from build123d import *

# Parameters (mm, degrees)
F0_R     = 22
F1_DEPTH = 6
F2_R     = 1.75
F3_DEPTH = 6.001
F4_R     = 5.5
F5_DEPTH = 4
F6_R     = 9
F7_DEPTH = 40
F8_R     = 5
F9_DEPTH = 35


with BuildPart() as f1:
    # F0 (on Front) → F1 (new body)
    with BuildSketch(Plane.XZ):
        Circle(F0_R)
    extrude(amount=F1_DEPTH)

    # F2 (on face) → F3 (cut, through all)
    with BuildSketch(Plane.XZ.offset(6)):
        with Locations((-8.301622, -8.665049)):
            Circle(F2_R)
        with Locations((8.665049, -8.301622)):
            Circle(F2_R)
        with Locations((-8.665049, 8.301622)):
            Circle(F2_R)
        with Locations((7.944154, 8.99391)):
            Circle(F2_R)
    extrude(amount=-F3_DEPTH, mode=Mode.SUBTRACT)

    # F4 (on face) → F5 (cut)
    with BuildSketch(Plane.XZ.offset(6)):
        Circle(F4_R)
    extrude(amount=-F5_DEPTH, mode=Mode.SUBTRACT)

    # F6 (on face) → F7 (join)
    with BuildSketch(Plane(origin=(0, 0, 0), x_dir=(-1, 0, 0), z_dir=(0, 1, 0))):
        Circle(F6_R)
    extrude(amount=F7_DEPTH)

    # F8 (on face) → F9 (cut)
    with BuildSketch(Plane(origin=(0, 40, 0), x_dir=(-1, 0, 0), z_dir=(0, 1, 0))):
        Circle(F8_R)
    extrude(amount=-F9_DEPTH, mode=Mode.SUBTRACT)


solid = f1.part
Source: CAD feature listing. Evaluate the final solid. Frame: model axes, mm. A direction names the side the tool comes from. Coordinates: 2 decimals unless noted, no trailing zeros. Loops run counter-clockwise (first coordinate to the right, second up) from the corner with the lowest first, then second, coordinate; pieces in that order, holes last. Notation, with made-up numbers: (5.25, 87) - (60.25, 87) arc R35 ccw to (60.25, 125) - close; hole circle Ø3 at (46.25, 28). An arc over 180 degrees is marked (long way). One line per question, with ' | ' between items.
1) Section C-C, the plane z = 0. Return loops of the section in (x, y), then the cut area to 3 significant figures.
Report:
outline: (-22, -6) - (-5.5, -6) - (-5.5, -2) - (5.5, -2) - (5.5, -6) - (22, -6) - (22, 0) - (9, 0) - (9, 40) - (5, 40) - (5, 5) - (-5, 5) - (-5, 40) - (-9, 40) - (-9, 0) - (-22, 0) - close | area: 590 mm²
2) First-contact query: P1, Ø12, axis at y = 32, z = -16.5, coming from the +X side; P2, Ø10, axis at x = -9, z = 17.5, coming from the +Y side; P3, Ø12, axis at x = -4, z = -12, coming from the +Y side; P4, Ø6, axis at y = 5, z = -5, coming from the +X side. Flat tips, straight axial feed; report the tip coordinate or a pass-through.
Report:
P1: passes through | P2: stops at y = 0 | P3: stops at y = 40 | P4: stops at x = 8.77
3) Section B-B, the plane y = 12. Return loops of the section in (x, z).
Report:
outline: circle Ø18 at (0, 0); hole circle Ø10 at (0, 0)
4) Pull-direction query (Z, two-part tool) for faces 1 (the face through (5, -6, -5)), 2 (the face through (-1.19, -4.03, -5.37)), 3 (the face through (8.437, -3.042, -6.567)), 4 (the face through (1.172, 19.72, 8.923)); classes: released by +Z, released by -Z, zero draft, split by the parting line, or undercut.
Report:
face 1: zero draft | face 2: undercut | face 3: undercut | face 4: split by the parting line
5) Section D-D, the plane x = 15. Return loops of the section in (y, z), then the cut area to 3 significant figures.
Report:
outline: (-6, -16.09) - (0, -16.09) - (0, 16.09) - (-6, 16.09) - close | area: 193 mm²
6) Set-up query: faces 5 (the face through (-0.3, 0, -9.5)), 6 (the face through (6.555, -3.042, 7.929)), 7 (the face through (0, -2, 0)). Return all of +Z, -Z, +X, -X, +Y, -Y with unobstructed straight access to the full face (end or side cutting, diameter ignored); none if empty.
Report:
face 5: +Y | face 6: +Y, -Y | face 7: -Y
7) Line query: line 1 along X through (y, z) = (-0.5, 9.5); line 2 along Y through (x, z) = (7, 6); line 3 along Z through (x, y) = (-3, 37.5). Output: solid intervals per line, ascending.
Report:
line 1: x = -19.84 to -9.94, -7.39 to 6.27, 9.62 to 19.84 | line 2: y = -6 to 0 | line 3: z = -8.49 to -4, 4 to 8.49
8) Section A-A, the plane x = 0. Return loops of the section in (y, z).
Report:
outline: (-6, -22) - (0, -22) - (0, -9) - (40, -9) - (40, -5) - (5, -5) - (5, 5) - (40, 5) - (40, 9) - (0, 9) - (0, 22) - (-6, 22) - (-6, 5.5) - (-2, 5.5) - (-2, -5.5) - (-6, -5.5) - close
